from build123d import *

# Parameters (mm, degrees)
F0_W      = 370
F0_H      = 450
F1_DEPTH  = 12
F2_R      = 3.5
F2_R_2    = 2.871219
F2_R_3    = 3
F3_DEPTH  = 12.001
F4_R      = 5
F5_R      = 7.5
F6_DEPTH  = 5
F7_R      = 2.5
F7_R_2    = 2
F8_DEPTH  = 30
F9_R      = 5
F10_DEPTH = 12.001


with BuildPart() as f1:
    # F0 (on Top) → F1 (new body)
    with BuildSketch(Plane.XY):
        Rectangle(F0_W, F0_H)
    extrude(amount=F1_DEPTH)

    # F2 (on Top) → F3 (cut, through all)
    with BuildSketch(Plane.XY):
        with Locations((-172, 106.5)):
            Circle(F2_R)
        with Locations((-172, 0)):
            Circle(F2_R)
        with Locations((-172, -332.140073)):
            Circle(F2_R_2)
        with Locations((60, 106.5)):
            Circle(F2_R)
        with Locations((60, 0)):
            Circle(F2_R)
        with Locations((60, -212)):
            Circle(F2_R)
        with Locations((60, 212)):
            Circle(F2_R)
        with Locations((-172, 212)):
            Circle(F2_R)
        with Locations((-172, -106.5)):
            Circle(F2_R)
        with Locations((-172, -212)):
            Circle(F2_R)
        with Locations((60, -106.5)):
            Circle(F2_R)
        with Locations((-55, 212)):
            Circle(F2_R)
        with Locations((-55, -212)):
            Circle(F2_R)
        with Locations((-55, -106.5)):
            Circle(F2_R)
        with Locations((-55, 106.5)):
            Circle(F2_R)
        with Locations((160, -165)):
            Circle(F2_R_3)
        with Locations((160, 165)):
            Circle(F2_R_3)
        with Locations((95, -165)):
            Circle(F2_R_3)
        with Locations((95, 165)):
            Circle(F2_R_3)
        with Locations((-55, 195)):
            Circle(F2_R)
        with Locations((-55, -195)):
            Circle(F2_R)
    extrude(amount=F3_DEPTH, mode=Mode.SUBTRACT)

    # F4
    f4_edges = [f1.edges().sort_by_distance(p)[0] for p in [
        (-185, -225, 6),
        (185, -225, 6),
        (185, 225, 6),
        (-185, 225, 6),
    ]]
    fillet(f4_edges, radius=F4_R)

    # F5 (on face) → F6 (cut)
    with BuildSketch(Plane.XY.offset(12)):
        with Locations((-172, 212)):
            Circle(F5_R)
        with Locations((-55, 212)):
            Circle(F5_R)
        with Locations((60, 212)):
            Circle(F5_R)
        with Locations((60, 106.5)):
            Circle(F5_R)
        with Locations((-55, 106.5)):
            Circle(F5_R)
        with Locations((-172, 106.5)):
            Circle(F5_R)
        with Locations((-172, 0)):
            Circle(F5_R)
        with Locations((60, 0)):
            Circle(F5_R)
        with Locations((-172, -106.5)):
            Circle(F5_R)
        with Locations((-55, -106.5)):
            Circle(F5_R)
        with Locations((60, -106.5)):
            Circle(F5_R)
        with Locations((60, -212)):
            Circle(F5_R)
        with Locations((-55, -212)):
            Circle(F5_R)
        with Locations((-172, -212)):
            Circle(F5_R)
        with Locations((-55, 195)):
            Circle(F5_R)
        with Locations((-55, -195)):
            Circle(F5_R)
    extrude(amount=-F6_DEPTH, mode=Mode.SUBTRACT)

    # F7 (on face) → F8 (cut)
    with BuildSketch(Plane.YZ.offset(185)):
        with Locations((100, 5)):
            Circle(F7_R)
        with Locations((200, 5)):
            Circle(F7_R)
        with Locations((-200, 5)):
            Circle(F7_R)
        with Locations((-100, 5)):
            Circle(F7_R)
        with Locations((0, 5)):
            Circle(F7_R)
        with Locations((150, 5)):
            Circle(F7_R_2)
        with Locations((-150, 5)):
            Circle(F7_R_2)
    extrude(amount=-F8_DEPTH, mode=Mode.SUBTRACT)

    # F9 (on Top) → F10 (cut, through all)
    with BuildSketch(Plane.XY):
        with Locations((-125, 125)):
            Circle(F9_R)
        with Locations((125, 125)):
            Circle(F9_R)
        with Locations((-125, -125)):
            Circle(F9_R)
        with Locations((125, -125)):
            Circle(F9_R)
    extrude(amount=F10_DEPTH, mode=Mode.SUBTRACT)


solid = f1.part
The listing builds one solid part. Answer for the finished solid, in the listing's coordinates (mm). A direction names the side the tool comes from. Give positions to 0.01 mm unless a question says otherwise; leave off trailing zeros. Order: outer loops, then holes, each group sorted by start corner. A loop starts at its lowest first (then second) coordinate and runs counter-clockwise, first axis right, second up. Notation, with made-up numbers: (-31.75, 46.5) - (27.25, 46.5) arc R31 ccw to (27.25, 82.5) - close; hole circle Ø7 at (13, 75.25). An arc over 180 degrees is marked (long way). Use one line per item in the form item = value.
1) Find section B-B on x = -125. Determine the outline of the cut face in (y, z).
Verdict:
outline = (-225, 0) - (-130, 0) - (-130, 12) - (-225, 12) - close; (-120, 0) - (120, 0) - (120, 12) - (-120, 12) - close; (130, 0) - (225, 0) - (225, 12) - (130, 12) - close
2) For faces 1 (the flat face through (58.2, -3.2, 7)), 2 (the flat face through (-3, -225, 6)), determine the directions among +Z, -Z, +X, -X, +Y, -Y from which every point of the face is accessible in a straight line to the end or side of a thin tool.
Verdict:
face_1 = +Z
face_2 = +Z, -Z, +X, -X, -Y
3) Consider probe 1 along Y at (x, z) = (-172, 2.75); probe 2 along X at (y, z) = (106.5, 3.5); probe 3 along X at (y, z) = (125, 6.5). Determine where each line is inside the solid, lowest interval first. Write a range as [from, to].
Verdict:
probe_1 = [-225, -215.5], [-208.5, -110], [-103, -3.5], [3.5, 103], [110, 208.5], [215.5, 225]
probe_2 = [-185, -175.5], [-168.5, -58.5], [-51.5, 56.5], [63.5, 185]
probe_3 = [-185, -130], [-120, 120], [130, 185]
4) Each of these flat-tipped pins is pushed along its axis until it touches: pin 1 (5 mm diameter, centred on x = -120.5, y = 100, fed in from -Z); pin 2 (8 mm diameter, centred on x = -172, y = -106.5, fed in from +Z); pin 3 (1.5 mm diameter, centred on y = 101, z = 6, fed in from +X). Where does it stop, or does it pass through?
Verdict:
pin_1 = 0
pin_2 = 7
pin_3 = 155
5) Find section C-C on z = 9.75. Give the number of separate pieces and of enclosed holes in the cut face, and give its area (3 significant figures).
Verdict:
separate_pieces = 1
enclosed_holes = 24
area = 163,000 mm^2
6) The mould has two halves that part along X. Classify faces 3 (the cylindrical face through (-55.976, 202.436, 9.535)), 4 (the flat face through (-3, 3, 12)): released by +X, released by -X, zero draft, split by the parting line, or undercut.
Verdict:
face_3 = undercut
face_4 = zero draft
7) Find section A-A on y = -125. Determine the outline of the cut face in (x, z), and give its area (3 significant figures).
Verdict:
outline = (-185, 0) - (-130, 0) - (-130, 12) - (-185, 12) - close; (-120, 0) - (120, 0) - (120, 12) - (-120, 12) - close; (130, 0) - (185, 0) - (185, 12) - (130, 12) - close
area = 4,200 mm^2
